from build123d import *

# Parameters (mm, degrees)
F1_DEPTH = 3
F2_DEPTH = 2
F3_R     = 2
F6_D     = 2


# Not quite as in the source:
# - a feature names something its author has since deleted; it is built from what else it names


with BuildPart() as f1:
    # F0 (on Top) → F1 (new body)
    with BuildSketch(Plane.XY):
        Polygon((-4.4, 4.75), (0, 4.75), (0, 8.75), (-14.8, 8.75), (-14.8, 0), (-8.8, 0), (-8.8, 4.75), align=None)
    extrude(amount=F1_DEPTH)

    # F0 (on Top) → F2 (join)
    with BuildSketch(Plane.XY):
        with BuildLine():
            ThreePointArc((-8.8, 0), (-7.5309776981, 3.2373793414), (-4.4, 4.75))
            Line((-4.4, 4.75), (-8.8, 4.75))
            Line((-8.8, 4.75), (-8.8, 0))
        make_face()
    extrude(amount=F2_DEPTH)

    # F3
    f3_edges = [f1.edges().sort_by_distance(p)[0] for p in [
        (-14.8, 8.75, 1.5),
        (-8.8, 4.75, 2.5),
    ]]
    fillet(f3_edges, radius=F3_R)

    # F4: F1 across face


with BuildPart() as f1_1:
    add(f1.part)
    add(f1.part.mirror(Plane(origin=(-11.8, 0, 1.5), x_dir=(1, 0, 0), z_dir=(0, -1, 0))))

    # F6 (through all)
    with Locations(Plane.XY.offset(3)):
        with Locations((-11.1, 0)):
            Hole(F6_D / 2)

    # F7: F1 across face


with BuildPart() as f1_2:
    add(f1_1.part)
    add(f1_1.part.mirror(Plane(origin=(0, 6.75, 1.5), x_dir=(0, 1, 0), z_dir=(1, 0, 0))))


solid = f1_2.part
The model under review builds one solid part; all positions refer to its coordinate system, in mm. A direction names the side the tool comes from. Round coordinates to 2 decimals unless told otherwise and drop trailing zeros. Loops run counter-clockwise (first coordinate to the right, second up) from the corner with the lowest first, then second, coordinate; pieces in that order, holes last. Notation, with made-up numbers: (68, 21) -> (72, 21) arc R24 cw to (72, 45) -> close; hole circle Ø10 at (13, 79). An arc over 180 degrees is marked (long way). Return JSON: item names as keys, results as strings.
(1) For pin 1 (2.5 mm diameter, centred on x = -11.1, y = 0, fed in from -Z); pin 2 (3.5 mm diameter, centred on x = -7, y = -1.5, fed in from +Z), all flat-tipped, find the tip position at first contact; note any pin that passes through.
Solved:
{"pin 1": "z = 0", "pin 2": "z = 2"}
(2) Add section C-C on y = -4.25. Write out the cut boundary in (x, z).
Solved:
{"outline": "(-14.8, 0) -> (-6.19, 0) -> (-6.19, 2) -> (-8.12, 2) -> (-8.12, 3) -> (-14.8, 3) -> close; (6.19, 0) -> (14.8, 0) -> (14.8, 3) -> (8.12, 3) -> (8.12, 2) -> (6.19, 2) -> close"}
(3) Add section D-D on x = 2.5. Write out the cut boundary in (y, z).
Solved:
{"outline": "(-8.75, 0) -> (-4.75, 0) -> (-4.75, 3) -> (-8.75, 3) -> close; (4.75, 0) -> (8.75, 0) -> (8.75, 3) -> (4.75, 3) -> close"}
(4) For faces 1 (the flat face through (-8.8, 0, 2.5)), 2 (the cylindrical face through (12.024, -0.383, 1.479)), list the 3-axis set-ups (+Z, -Z, +X, -X, +Y, -Y) from which the entire face can be reached by the end or side of a thin tool; tool diameter is ignored.
Solved:
{"face 1": "+Z", "face 2": "+Z, -Z"}
(5) For line 1 (Y direction, x = 0.75, z = 2.1); line 2 (X direction, y = -1.75, z = 2.2); line 3 (Y direction, x = -11, z = 1.65), list the stretches that pass through material, from the lowest coordinate up.
Solved:
{"line 1": "-8.75 to -4.75, 4.75 to 8.75", "line 2": "-14.8 to -8.8, 8.8 to 14.8", "line 3": "-8.75 to -0.99, 0.99 to 8.75"}
(6) Add section A-A on x = -11.1. Write out the cut boundary in (y, z).
Solved:
{"outline": "(-8.75, 0) -> (-1, 0) -> (-1, 3) -> (-8.75, 3) -> close; (1, 0) -> (8.75, 0) -> (8.75, 3) -> (1, 3) -> close"}
(7) The part is to be moulded in two halves that separate along Y. For faces 3 (the flat face through (0, -8.75, 1)), 4 (the flat face through (-14.8, 0, 1)), 5 (the flat face through (-8, 3, 2)), 6 (the flat face through (0, 4.75, 2)), say which applies: released by +Y, released by -Y, zero draft, split by the parting line, or undercut.
Solved:
{"face 3": "released by -Y", "face 4": "zero draft", "face 5": "undercut", "face 6": "undercut"}
(8) Add section B-B on z = 0.95. Write out the cut boundary in (x, y), plus the area to 3 significant figures.
Solved:
{"outline": "(-14.8, -6.75) arc R2 ccw to (-12.8, -8.75) -> (12.8, -8.75) arc R2 ccw to (14.8, -6.75) -> (14.8, 6.75) arc R2 ccw to (12.8, 8.75) -> (-12.8, 8.75) arc R2 ccw to (-14.8, 6.75) -> close; hole circle Ø2 at (-11.1, 0); hole (-4.4, -4.75) -> (4.4, -4.75) arc R4.76 ccw to (4.4, 4.75) -> (-4.4, 4.75) arc R4.76 ccw to start; hole circle Ø2 at (11.1, 0)", "area": "360 mm2"}
